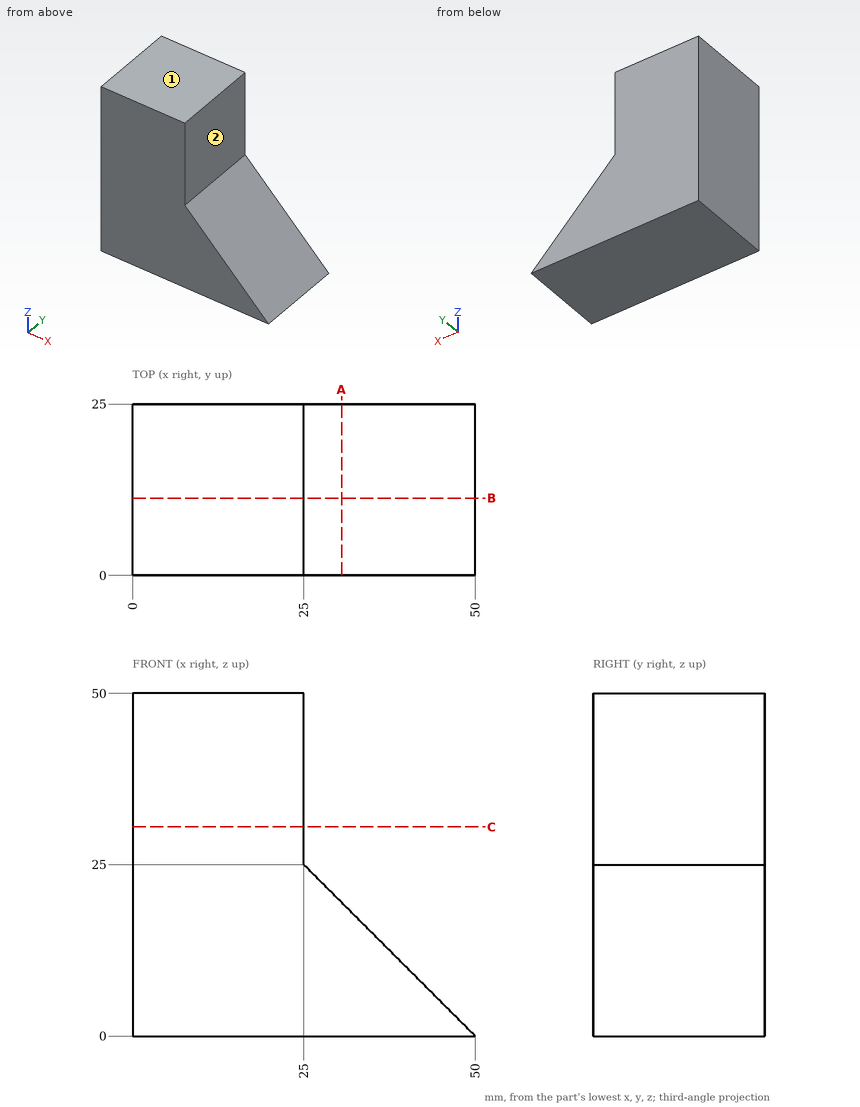
Geometry: see drawing. Coordinates: mm, zero at the bounding-box minimum. A direction names the side the tool comes from. Give positions to 0.01 mm unless a question says otherwise; leave off trailing zeros. Loops run counter-clockwise (first coordinate to the right, second up) from the corner with the lowest first, then second, coordinate; pieces in that order, holes last. Notation, with made-up numbers: (-31, 38.5) -> (-20, 38.5) arc R33 cw to (-20, 75.5) -> close; hole circle Ø11 at (-9, 65). An arc over 180 degrees is marked (long way). Answer as a JSON object with one key per item and string values. Group by question number.
Item 1: Pin query (flat end, axial travel): P1, Ø3, axis at y = 8.5, z = 43.5, coming from the -X side; P2, Ø7.5, axis at y = 9, z = 35.5, coming from the +X side; P3, Ø4, axis at y = 6.5, z = 14.5, coming from the +X side. Return the tip coordinate at first contact, or that it passes through.
Item 2: Cut plane C-C, the plane z = 30.5. Return the cut outline in (x, y).
Item 3: Reachability of the marked faces 1 and 2 from +Z, -Z, +X, -X, +Y, -Y: full face, straight path, thin tool, end or side. Return the list, or none.
Item 4: Cut plane A-A, the plane x = 30.5. Return the cut outline in (y, z), and give its area (4 significant figures).
Item 5: Cut plane B-B, the plane y = 11.25. Return the cut outline in (x, z), and give its area (3 significant figures).
Item 6: Line query: probe 1 along X at (y, z) = (8.5, 28); probe 2 along X at (y, z) = (8.5, 8); probe 3 along Z at (x, y) = (34, 23.5). Output: solid intervals per line, ascending.
Checks:
{
 "1": {"P1": "stops at x = 0", "P2": "stops at x = 25", "P3": "stops at x = 37.5"},
 "2": {"outline": "(0, 0) -> (25, 0) -> (25, 25) -> (0, 25) -> close"},
 "3": {"face 1": "+Z, +X, -X, +Y, -Y", "face 2": "+Z, +X, +Y, -Y"},
 "4": {"outline": "(0, 0) -> (25, 0) -> (25, 19.5) -> (0, 19.5) -> close", "area": "487.5 mm²"},
 "5": {"outline": "(0, 0) -> (50, 0) -> (25, 25) -> (25, 50) -> (0, 50) -> close", "area": "1,560 mm²"},
 "6": {"probe 1": "x = 0 to 25", "probe 2": "x = 0 to 42", "probe 3": "z = 0 to 16"}
}
